from build123d import *

# Parameters (mm, degrees)
F1_DEPTH = 25.4
F2_T     = -2.54
F3_R     = 3.175
F4_DEPTH = 25.4


with BuildPart() as f1:
    # F0 (on Top) → F1 (new body)
    with BuildSketch(Plane.XY):
        Polygon((-58.3186791779, 0), (-29.159339589, -16.8351525611), (-29.159339589, -50.5054576833), (0, -33.6703051222), (29.159339589, -50.5054576833), (29.159339589, -16.8351525611), (58.3186791779, 0), (29.159339589, 16.8351525611), (29.159339589, 50.5054576833), (0, 33.6703051222), (-29.159339589, 50.5054576833), (-29.159339589, 16.8351525611), align=None)
    extrude(amount=F1_DEPTH)

    # F2
    f2_openings = [f1.faces().sort_by_distance(p)[0] for p in [
        (0, 0, 25.4),
    ]]
    offset(amount=F2_T, openings=f2_openings, kind=Kind.INTERSECTION)

    # F3 (on face) → F4 (cut)
    with BuildSketch(Plane.XY.offset(2.54)):
        with Locations((5.08, 8.7988181024)):
            Circle(F3_R)
        with Locations((10.16, 0)):
            Circle(F3_R)
        with Locations((5.08, -8.7988181024)):
            Circle(F3_R)
        with Locations((-5.08, -8.7988181024)):
            Circle(F3_R)
        with Locations((-10.16, 0)):
            Circle(F3_R)
        with Locations((-5.08, 8.7988181024)):
            Circle(F3_R)
    extrude(amount=-F4_DEPTH, mode=Mode.SUBTRACT)


solid = f1.part
Work out the finished part from the listing and answer in its coordinate system (mm). A direction names the side the tool comes from. Coordinates: 2 decimals unless noted, no trailing zeros. Loops run counter-clockwise (first coordinate to the right, second up) from the corner with the lowest first, then second, coordinate; pieces in that order, holes last. Notation, with made-up numbers: M 11.25,57.5 L 60.25,57.5 A9 ccw 60.25,66.5 Z; hole C -3.5,-6.5 d2. An arc over 180 degrees is marked long. Answer in a Markdown table with one row per item. Add a question column.
1. The mould has two halves that part along Y. Classify faces 5 (the flat face through (-43.94, -8.3, 12.52)), 6 (the flat face through (29.159, 33, 13)), 7 (the flat face through (-26.619, -31, 14)), 8 (the flat face through (-26.619, 31, 14)): pulls with the +Y half, pulls with the -Y half, needs draft (parallel to the pull), parting line crosses it, or undercut.
2. Flat-ended cylindrical pins translate along their axes: P1, Ø7.5, axis at y = -29.5, z = 11, coming from the +X side; P2, Ø1, axis at x = -20, z = 8, coming from the +Y side; P3, Ø5, axis at x = -43, z = 5, coming from the +Y side; P4, Ø10, axis at x = -10.16, y = 0, coming from the -Z side. Find the tip coordinate at first contact, or state that the pin passes through.
3. Find section D-D, the plane y = 37. Write down the section's boundary in (x, z).
4. Consider L1, parallel to X at y = -21, z = 13.5; L2, parallel to X at y = 43.5, z = 10; L3, parallel to X at y = 37, z = 7.5. Determine where each line is inside the solid, lowest interval first.
5. Find section B-B, the plane z = 11.5. Write down the section's boundary in (x, y).
6. Find section A-A, the plane x = 5.08. Write down the section's boundary in (y, z).
7. A tool of negligible diameter and unlimited length cuts with its end or side. For faces 1 (the flat face through (-39.743, 7.792, 13.81)), 2 (the flat face through (14.784, 42.206, 12.522)), 3 (the flat face through (-29.159, -33, 13)), 4 (the flat face through (-43.53, 8.54, 12.52)), from which of +Z, -Z, +X, -X, +Y, -Y can it reach the whole face along a straight path? Write none if from no direction.
8. Find section C-C, the plane x = -10.16. Write down the section's boundary in (y, z) (3 decimals), then the cut area to 3 significant figures.
Reported:
| question | item | result |
|---|---|---|
| 1 | face 5 | pulls with the -Y half |
| 1 | face 6 | needs draft |
| 1 | face 7 | undercut |
| 1 | face 8 | undercut |
| 2 | P1 | stops at x = 29.16 |
| 2 | P2 | stops at y = 45.51 |
| 2 | P3 | stops at y = 10.29 |
| 2 | P4 | stops at z = 0 |
| 3 | outline | M -29.16,0 L -5.77,0 L -5.77,25.4 L -10.85,25.4 L -10.85,2.54 L -26.62,2.54 L -26.62,25.4 L -29.16,25.4 Z; M 5.77,0 L 29.16,0 L 29.16,25.4 L 26.62,25.4 L 26.62,2.54 L 10.85,2.54 L 10.85,25.4 L 5.77,25.4 Z |
| 4 | L1 | x = -29.16 to -26.62, 26.62 to 29.16 |
| 4 | L2 | x = -29.16 to -26.62, -22.11 to -17.03, 17.03 to 22.11, 26.62 to 29.16 |
| 4 | L3 | x = -29.16 to -26.62, -10.85 to -5.77, 5.77 to 10.85, 26.62 to 29.16 |
| 5 | outline | M -58.32,0 L -29.16,-16.84 L -29.16,-50.51 L 0,-33.67 L 29.16,-50.51 L 29.16,-16.84 L 58.32,0 L 29.16,16.84 L 29.16,50.51 L 0,33.67 L -29.16,50.51 L -29.16,16.84 Z; hole M -53.24,0 L -26.62,-15.37 L -26.62,-46.11 L 0,-30.74 L 26.62,-46.11 L 26.62,-15.37 L 53.24,0 L 26.62,15.37 L 26.62,46.11 L 0,30.74 L -26.62,46.11 L -26.62,15.37 Z |
| 6 | outline | M -36.6,0 L -11.97,0 L -11.97,2.54 L -33.67,2.54 L -33.67,25.4 L -36.6,25.4 Z; M -5.62,0 L 5.62,0 L 5.62,2.54 L -5.62,2.54 Z; M 11.97,0 L 36.6,0 L 36.6,25.4 L 33.67,25.4 L 33.67,2.54 L 11.97,2.54 Z |
| 7 | face 1 | +Z |
| 7 | face 2 | +Z, -Z, +Y |
| 7 | face 3 | +Z, -Z, -X, -Y |
| 7 | face 4 | +Z, -Z, -X, +Y |
| 8 | outline | M -39.536,0 L -3.175,0 L -3.175,2.54 L -36.603,2.54 L -36.603,25.4 L -39.536,25.4 Z; M 3.175,0 L 39.536,0 L 39.536,25.4 L 36.603,25.4 L 36.603,2.54 L 3.175,2.54 Z |
| 8 | area | 319 mm^2 |
